The model under review builds one solid part; all positions refer to its coordinate system, in mm. Face numbers are marked on the shaded views. A direction names the side the tool comes from. Coordinates: 2 decimals unless noted, no trailing zeros. Write each loop counter-clockwise with the first axis right and the second up, starting at its lowest first coordinate (ties: lowest second). Pieces come first, ordered by that corner, then holes.
1) For line 1 (Y direction, x = -0.75, z = 5); line 2 (Y direction, x = 0, z = 2.25); line 3 (Y direction, x = -1.5, z = 5.5), list the stretches that pass through material, from the lowest coordinate up.
2) Machinability: for the marked faces 1, 2 and 3, which of the approach directions +Z, -Z, +X, -X, +Y, -Y give a long, thin tool a straight path to every point of the face, cutting with its end or side? Answer none if there is none.
3) Add section B-B, the plane x = 0. Give the number of separate pieces and of enclosed holes in the cut face, then the cut area to 3 significant figures.
4) For P1, Ø4.5, axis at x = 0, y = -5.93, coming from the -Z side; P2, Ø3, axis at y = 3.5, z = 4, coming from the -X side; P3, Ø3.5, axis at x = 0, y = 0, coming from the -Z side; P4, Ø1.5, axis at y = 6, z = 5.5, coming from the -X side, all flat-tipped, find the tip position at first contact; note any pin that passes through.
5) Mouldability with a two-part tool opening along X and no side actions: class the marked faces 4, 5 and 6 as released by +X, released by -X, zero draft, split by the parting line, or undercut.
6) Add section A-A, the plane z = 0.5. State the section outline as (x, y) points, then the cut area to 3 significant figures.
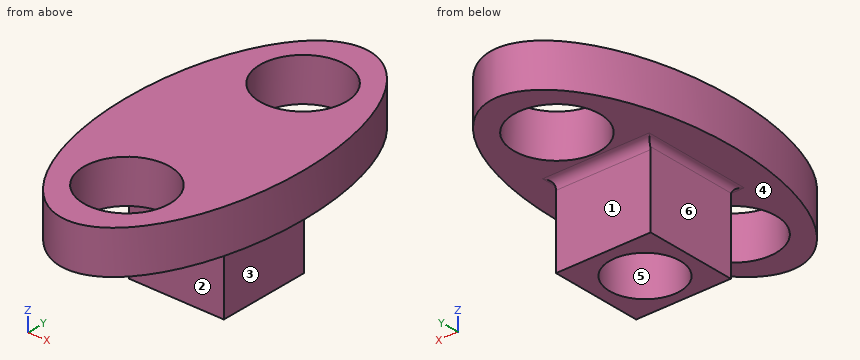
from build123d import *
from OCP.BRepFilletAPI import BRepFilletAPI_MakeFillet

# Parameters (mm, degrees)
ESQUISSE4_W             = 5.5
ESQUISSE4_H             = 5.4
BOSS_EXTRU_2_DEPTH      = 4.7
ESQUISSE5_RX            = 10
ESQUISSE5_RY            = 5.046155586
ESQUISSE5_R             = 2.5
BOSS_EXTRU_4_DEPTH      = 2.5
ESQUISSE6_R             = 2.05
ENL_V_MAT_EXTRU_1_DEPTH = 4.32
CONG_1_R1               = 0.2
CONG_1_R2               = 0.35
CONG_1_R3               = 0.5


with BuildPart() as part:
    # Esquisse4 → Boss.-Extru.2 (new body)
    with BuildSketch(Plane.XY):
        with Locations((0.05, 0.05)):
            Rectangle(ESQUISSE4_W, ESQUISSE4_H)
    extrude(amount=BOSS_EXTRU_2_DEPTH)

    # Esquisse5 → Boss.-Extru.4 (add)
    with BuildSketch(Plane.XY.offset(4.7)):
        with Locations(Location((0, 0), (0, 0, 90))):
            Ellipse(ESQUISSE5_RX, ESQUISSE5_RY)
        with Locations((0, 5.93)):
            Circle(ESQUISSE5_R, mode=Mode.SUBTRACT)
        with Locations((0, -5.93)):
            Circle(ESQUISSE5_R, mode=Mode.SUBTRACT)
    extrude(amount=BOSS_EXTRU_4_DEPTH)

    # Esquisse6 → Enlèv. mat.-Extru.1 (cut)
    with BuildSketch(Plane(origin=(0, 0, 0), x_dir=(-1, 0, 0), z_dir=(0, 0, -1))):
        Circle(ESQUISSE6_R)
    extrude(amount=-ENL_V_MAT_EXTRU_1_DEPTH, mode=Mode.SUBTRACT)

    # Congé1: one fillet with a radius per group of edges: ONE call of the kernel's fillet builder (fillet() takes one radius for all edges)
    cong_1_edges_1 = [part.edges().sort_by_distance(p)[0] for p in [
        (2.05, 0, 4.32),
    ]]
    cong_1_edges_2 = [part.edges().sort_by_distance(p)[0] for p in [
        (2.8, 0.05, 4.7),
        (-2.7, 0.05, 4.7),
    ]]
    cong_1_edges_3 = [part.edges().sort_by_distance(p)[0] for p in [
        (0.05, 2.75, 4.7),
        (0.05, -2.65, 4.7),
    ]]
    cong_1 = BRepFilletAPI_MakeFillet(part.part.solid().wrapped)
    for e in cong_1_edges_1:
        cong_1.Add(CONG_1_R1, e.wrapped)
    for e in cong_1_edges_2:
        cong_1.Add(CONG_1_R2, e.wrapped)
    for e in cong_1_edges_3:
        cong_1.Add(CONG_1_R3, e.wrapped)
    add(Compound.cast(cong_1.Shape()), mode=Mode.REPLACE)


solid = part.part
Geometry results:
1. line 1: y = -9.89 to -8.31, -3.55 to 3.55, 8.31 to 9.89
1. line 2: y = -2.65 to -2.05, 2.05 to 2.75
1. line 3: y = -9.55 to -7.93, -3.93 to 3.93, 7.93 to 9.55
2. face 1: -Z, +X, -X, +Y
2. face 2: -Z, +X, -X, -Y
2. face 3: -Z, +X, +Y, -Y
3. separate pieces: 3
3. enclosed holes: 0
3. area: 32.8 mm2
4. P1: passes through
4. P2: stops at x = -4.93
4. P3: stops at z = 4.32
4. P4: stops at x = -4.29
5. face 4: zero draft
5. face 5: undercut
5. face 6: released by -X
6. outline: (-2.7, -2.65) - (2.8, -2.65) - (2.8, 2.75) - (-2.7, 2.75) - close; hole circle Ø4.1 at (0, 0)
6. area: 16.5 mm2
